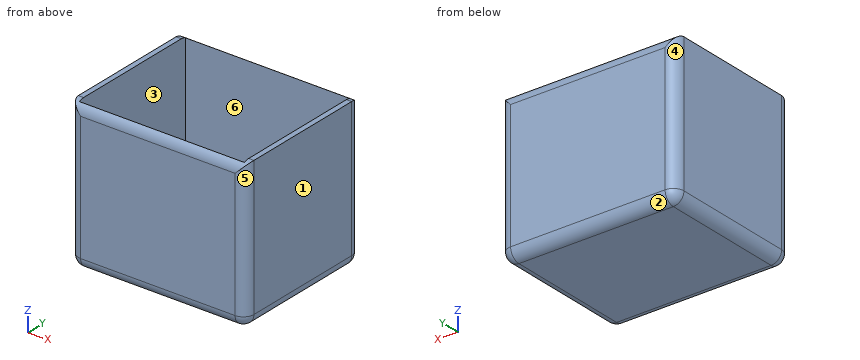
from build123d import *

# Parameters (mm, degrees)
F0_W         = 84.3196734786
F0_H         = 70.0790211558
F1_DEPTH     = 71.12
F2_T         = -2.54
F3_T1_DEPTH  = 78.74
F3_T3_DEPTH  = 109.7196734786
F3_T5_DEPTH  = 74.1596734786
F3_T7_DEPTH  = 59.9190211558
F3_S11_W     = 5.08
F3_S11_H     = 5.08
F3_T12_DEPTH = 5.08
F3_S17_W     = 5.08
F3_S17_H     = 5.08
F3_T18_DEPTH = 5.08
F3_S23_W     = 5.08
F3_S23_H     = 5.08
F3_T24_DEPTH = 5.08
F3_S29_W     = 5.08
F3_S29_H     = 5.08
F3_T30_DEPTH = 5.08


# Not quite as in the source:
# - a fillet or chamfer that OpenCascade refuses, or shapes differently, is made with other operations: its cross-section is extruded or revolved along the edge and cut away or added


with BuildPart() as f1:
    # F0 (on Top) → F1 (new body)
    with BuildSketch(Plane.XY):
        with Locations((-0.5621314049, -4.3096728623)):
            Rectangle(F0_W, F0_H)
    extrude(amount=F1_DEPTH)

    # F2
    f2_openings = [f1.faces().sort_by_distance(p)[0] for p in [
        (-0.562131, -4.309673, 71.12),
    ]]
    offset(amount=F2_T, openings=f2_openings)

    # F3: fillet of radius 5.08 on 10 edges, made by hand

    # F3_s2 → F3_t1 (cut)
    with BuildSketch(Plane.XY.offset(5.08)):
        with BuildLine():
            ThreePointArc((36.5177053344, -39.3491834402), (40.1098077829, -37.8612858886), (41.5977053344, -34.2691834402))
            Line((41.5977053344, -34.2691834402), (41.5977053344, -39.3491834402))
            Line((41.5977053344, -39.3491834402), (36.5177053344, -39.3491834402))
        make_face()
        with BuildLine():
            ThreePointArc((-42.7219681442, -34.2691834402), (-41.2340705926, -37.8612858886), (-37.6419681442, -39.3491834402))
            Line((-37.6419681442, -39.3491834402), (-42.7219681442, -39.3491834402))
            Line((-42.7219681442, -39.3491834402), (-42.7219681442, -34.2691834402))
        make_face()
        with BuildLine():
            ThreePointArc((36.5177053344, 30.7298377156), (40.1098077829, 29.2419401641), (41.5977053344, 25.6498377156))
            Line((41.5977053344, 25.6498377156), (41.5977053344, 30.7298377156))
            Line((41.5977053344, 30.7298377156), (36.5177053344, 30.7298377156))
        make_face()
        with BuildLine():
            ThreePointArc((-37.6419681442, 30.7298377156), (-41.2340705926, 29.2419401641), (-42.7219681442, 25.6498377156))
            Line((-42.7219681442, 25.6498377156), (-42.7219681442, 30.7298377156))
            Line((-42.7219681442, 30.7298377156), (-37.6419681442, 30.7298377156))
        make_face()
    extrude(amount=F3_T1_DEPTH, mode=Mode.SUBTRACT)

    # F3_s4 → F3_t3 (cut)
    with BuildSketch(Plane.YZ.offset(-55.4219681442)):
        with BuildLine():
            ThreePointArc((30.7298377156, 66.04), (29.2419401641, 69.6321024484), (25.6498377156, 71.12))
            Line((25.6498377156, 71.12), (30.7298377156, 71.12))
            Line((30.7298377156, 71.12), (30.7298377156, 66.04))
        make_face()
        with BuildLine():
            ThreePointArc((-39.3491834402, 66.04), (-37.8612858886, 69.6321024484), (-34.2691834402, 71.12))
            Line((-34.2691834402, 71.12), (-39.3491834402, 71.12))
            Line((-39.3491834402, 71.12), (-39.3491834402, 66.04))
        make_face()
    extrude(amount=F3_T3_DEPTH, mode=Mode.SUBTRACT)

    # F3_s6 → F3_t5 (cut)
    with BuildSketch(Plane.YZ.offset(-37.6419681442)):
        with BuildLine():
            ThreePointArc((30.7298377156, 5.08), (29.2419401641, 1.4878975516), (25.6498377156, 0))
            Line((25.6498377156, 0), (30.7298377156, 0))
            Line((30.7298377156, 0), (30.7298377156, 5.08))
        make_face()
        with BuildLine():
            ThreePointArc((-39.3491834402, 5.08), (-37.8612858886, 1.4878975516), (-34.2691834402, 0))
            Line((-34.2691834402, 0), (-39.3491834402, 0))
            Line((-39.3491834402, 0), (-39.3491834402, 5.08))
        make_face()
    extrude(amount=F3_T5_DEPTH, mode=Mode.SUBTRACT)

    # F3_s8 → F3_t7 (cut)
    with BuildSketch(Plane.XZ.offset(-25.6498377156)):
        with BuildLine():
            ThreePointArc((41.5977053344, 5.08), (40.1098077829, 1.4878975516), (36.5177053344, 0))
            Line((36.5177053344, 0), (41.5977053344, 0))
            Line((41.5977053344, 0), (41.5977053344, 5.08))
        make_face()
        with BuildLine():
            ThreePointArc((-42.7219681442, 5.08), (-41.2340705926, 1.4878975516), (-37.6419681442, 0))
            Line((-37.6419681442, 0), (-42.7219681442, 0))
            Line((-42.7219681442, 0), (-42.7219681442, 5.08))
        make_face()
    extrude(amount=F3_T7_DEPTH, mode=Mode.SUBTRACT)


with BuildPart() as f3_tool10:
    # F3_s11 → F3_t12 (new body)
    with BuildSketch(Plane.XZ.offset(34.2691834402)):
        with Locations((39.0577053344, 2.54)):
            Rectangle(F3_S11_W, F3_S11_H)
    extrude(amount=F3_T12_DEPTH)

    # F3_s13 → F3_t14 (revolve, cut)
    with BuildSketch(Plane(origin=(36.5177053344, -34.2691834402, 5.08), x_dir=(-0.7071067812, 0, 0.7071067812), z_dir=(0.7071067812, 0, 0.7071067812))):
        with BuildLine():
            ThreePointArc((0, -5.08), (5.08, 0), (0, 5.08))
            Line((0, 5.08), (0, -5.08))
        make_face()
    revolve(axis=Axis((36.5177053344, -34.2691834402, 5.08), (0, -1, 0)), mode=Mode.SUBTRACT)


with BuildPart() as f1_1:
    add(f1.part)

    # F3_t9: cut F3_tool10
    add(f3_tool10.part, mode=Mode.SUBTRACT)


with BuildPart() as f3_tool16:
    # F3_s17 → F3_t18 (new body)
    with BuildSketch(Plane.YZ.offset(-37.6419681442)):
        with Locations((-36.8091834402, 2.54)):
            Rectangle(F3_S17_W, F3_S17_H)
    extrude(amount=-F3_T18_DEPTH)

    # F3_s19 → F3_t20 (revolve, cut)
    with BuildSketch(Plane(origin=(-37.6419681442, -34.2691834402, 5.08), x_dir=(0, 0.7071067812, 0.7071067812), z_dir=(0, -0.7071067812, 0.7071067812))):
        with BuildLine():
            ThreePointArc((0, -5.08), (5.08, 0), (0, 5.08))
            Line((0, 5.08), (0, -5.08))
        make_face()
    revolve(axis=Axis((-37.6419681442, -34.2691834402, 5.08), (-1, 0, 0)), mode=Mode.SUBTRACT)


with BuildPart() as f1_2:
    add(f1_1.part)

    # F3_t15: cut F3_tool16
    add(f3_tool16.part, mode=Mode.SUBTRACT)


with BuildPart() as f3_tool22:
    # F3_s23 → F3_t24 (new body)
    with BuildSketch(Plane.XZ.offset(-25.6498377156)):
        with Locations((39.0577053344, 2.54)):
            Rectangle(F3_S23_W, F3_S23_H)
    extrude(amount=-F3_T24_DEPTH)

    # F3_s25 → F3_t26 (revolve, cut)
    with BuildSketch(Plane(origin=(36.5177053344, 25.6498377156, 5.08), x_dir=(-0.7071067812, 0, 0.7071067812), z_dir=(-0.7071067812, 0, -0.7071067812))):
        with BuildLine():
            ThreePointArc((0, -5.08), (5.08, 0), (0, 5.08))
            Line((0, 5.08), (0, -5.08))
        make_face()
    revolve(axis=Axis((36.5177053344, 25.6498377156, 5.08), (0, 1, 0)), mode=Mode.SUBTRACT)


with BuildPart() as f1_3:
    add(f1_2.part)

    # F3_t21: cut F3_tool22
    add(f3_tool22.part, mode=Mode.SUBTRACT)


with BuildPart() as f3_tool28:
    # F3_s29 → F3_t30 (new body)
    with BuildSketch(Plane.XZ.offset(-25.6498377156)):
        with Locations((-40.1819681442, 2.54)):
            Rectangle(F3_S29_W, F3_S29_H)
    extrude(amount=-F3_T30_DEPTH)

    # F3_s31 → F3_t32 (revolve, cut)
    with BuildSketch(Plane(origin=(-37.6419681442, 25.6498377156, 5.08), x_dir=(0.7071067812, 0, 0.7071067812), z_dir=(-0.7071067812, 0, 0.7071067812))):
        with BuildLine():
            ThreePointArc((0, -5.08), (5.08, 0), (0, 5.08))
            Line((0, 5.08), (0, -5.08))
        make_face()
    revolve(axis=Axis((-37.6419681442, 25.6498377156, 5.08), (0, 1, 0)), mode=Mode.SUBTRACT)


with BuildPart() as f1_4:
    add(f1_3.part)

    # F3_t27: cut F3_tool28
    add(f3_tool28.part, mode=Mode.SUBTRACT)


solid = f1_4.part
The listing builds one solid part. Answer for the finished solid, in the listing's coordinates (mm). Face numbers are marked on the shaded views. A direction names the side the tool comes from. Coordinates: 2 decimals unless noted, no trailing zeros. Write each loop counter-clockwise with the first axis right and the second up, starting at its lowest first coordinate (ties: lowest second). Pieces come first, ordered by that corner, then holes. Notation, with made-up numbers: M 75.5,-20.75 L 122.5,-20.75 A14 cw 122.5,-11.75 Z; hole C 58,36.5 d8. An arc over 180 degrees is marked long. Put each result on its own line as item: value. Start each with the question number.
1. A flat-ended cylindrical pin translates along its axis: P1, Ø1, axis at x = -4, y = -7, coming from the +Z side. Find the tip coordinate at first contact, or state that the pin passes through.
2. For a pull along X with two mould halves and no side action, classify the marked faces 1, 2, 3 and 4 as pulls with the +X half, pulls with the -X half, needs draft (parallel to the pull), parting line crosses it, or undercut.
3. A cutting plane is placed at C-C on x = 22. Write down the section's boundary in (y, z), then the cut area to 3 significant figures.
4. Consider line 1 (Y direction, x = -16.5, z = 47.5); line 2 (X direction, y = -26, z = 21.5); line 3 (Z direction, x = -32, y = -26). Determine where each line is inside the solid, lowest interval first. Write a range as from..to.
5. A cutting plane is placed at B-B on y = -17.5. Write down the section's boundary in (x, z), then the cut area to 3 significant figures.
6. A cutting plane is placed at A-A on z = 11.5. Write down the section's boundary in (x, y).
7. Which of the six approach directions +Z, -Z, +X, -X, +Y, -Y give full straight-line access (tool end or side, diameter ignored) to the marked faces 5 and 6?
Resolved:
1. P1: stops at z = 2.54
2. face 1: pulls with the +X half
2. face 2: needs draft
2. face 3: undercut
2. face 4: pulls with the -X half
3. outline: M -39.35,5.08 A5.08 ccw -34.27,0 L 25.65,0 A5.08 ccw 30.73,5.08 L 30.73,66.04 A5.08 ccw 28.19,70.44 L 28.19,2.54 L -36.81,2.54 L -36.81,70.44 A5.08 ccw -39.35,66.04 Z
3. area: 505 mm2
4. line 1: y = -39.35..-36.81, 28.19..30.73
4. line 2: x = -42.72..-40.18, 39.06..41.6
4. line 3: z = 0..2.54
5. outline: M -42.72,5.08 A5.08 ccw -37.64,0 L 36.52,0 A5.08 ccw 41.6,5.08 L 41.6,71.12 L 39.06,71.12 L 39.06,2.54 L -40.18,2.54 L -40.18,71.12 L -42.72,71.12 Z
5. area: 551 mm2
6. outline: M -42.72,-34.27 A5.08 ccw -37.64,-39.35 L 36.52,-39.35 A5.08 ccw 41.6,-34.27 L 41.6,25.65 A5.08 ccw 36.52,30.73 L -37.64,30.73 A5.08 ccw -42.72,25.65 Z; hole M -40.18,-36.81 L 39.06,-36.81 L 39.06,28.19 L -40.18,28.19 Z
7. face 5: +Z, -Z, +X, -Y
7. face 6: +Z
